```python
from build123d import *

# Parameters (mm, degrees)
F0_W     = 125
F0_H     = 95
F0_H_2   = 40
F1_DEPTH = 102
F2_START = 46
F2_DEPTH = 86.07192
F3_W     = 24
F3_H     = 50
F4_DEPTH = 3


with BuildPart() as f1:
    # F0 (on Top) → F1 (new body)
    with BuildSketch(Plane.XY):
        with Locations((62.5, 47.5)):
            Rectangle(F0_W, F0_H)
        with Locations((62.5, 115)):
            Rectangle(F0_W, F0_H_2)
    extrude(amount=F1_DEPTH)

    # F0 (on Top) → F2 (cut)
    with BuildSketch(Plane.XY.offset(F2_START)):
        with Locations((62.5, 115)):
            Rectangle(F0_W, F0_H_2)
    extrude(amount=F2_DEPTH, mode=Mode.SUBTRACT)

    # F3 (on face) → F4 (join)
    with BuildSketch(Plane.XZ):
        with Locations((15.6, 48)):
            Rectangle(F3_W, F3_H)
    extrude(amount=F4_DEPTH)


solid = f1.part
```
Can you work these out from the model? Positions are in its coordinate system, mm. A direction names the side the tool comes from. Round coordinates to 2 decimals unless told otherwise and drop trailing zeros. Loops run counter-clockwise (first coordinate to the right, second up) from the corner with the lowest first, then second, coordinate; pieces in that order, holes last. Notation, with made-up numbers: (67, 58.25) -> (112, 58.25) arc R15 cw to (112, 71.25) -> close; hole circle Ø10 at (-22.75, 52). An arc over 180 degrees is marked (long way). One line per item, written item: value. Start each with the question number.
1. If we section it at A-A, the plane x = 10: Write out the boundary of the cut face in (y, z).
2. For faces 1 (the flat face through (62, 115, 46)), 2 (the flat face through (62, 68, 0)), which set-ups out of +Z, -Z, +X, -X, +Y, -Y let a thin tool reach every point of the face, with its end or its side?
3. For pin 1 (1.5 mm diameter, centred on y = -1.5, z = 36.5, fed in from +X); pin 2 (6 mm diameter, centred on y = 70, z = 22.5, fed in from -X); pin 3 (3.5 mm diameter, centred on x = 10, y = -2, fed in from -Z); pin 4 (1.5 mm diameter, centred on x = 51, z = 19, fed in from -Y), each with a flat end and sliding along its axis, tell me the tip position at first contact or that it passes through.
4. If we section it at C-C, the plane x = 117.5: Write out the boundary of the cut face in (y, z).
5. If we section it at D-D, the plane y = 99: Write out the boundary of the cut face in (x, z), then the cut area to 3 significant figures.
6. If I drill on probe 1 along Y at (x, z) = (15, 63); probe 2 along Z at (x, y) = (20.5, 107); probe 3 along Y at (x, z) = (15.5, 82.5), over which ranges is the centre line in solid material (lowest first)?
7. If we section it at B-B, the plane z = 28: Write out the boundary of the cut face in (x, y).
Calculated:
1. outline: (-3, 23) -> (0, 23) -> (0, 0) -> (135, 0) -> (135, 46) -> (95, 46) -> (95, 102) -> (0, 102) -> (0, 73) -> (-3, 73) -> close
2. face 1: +Z, +X, -X, +Y
2. face 2: -Z, +X, -X, +Y, -Y
3. pin 1: stops at x = 27.6
3. pin 2: stops at x = 0
3. pin 3: stops at z = 23
3. pin 4: stops at y = 0
4. outline: (0, 0) -> (135, 0) -> (135, 46) -> (95, 46) -> (95, 102) -> (0, 102) -> close
5. outline: (0, 0) -> (125, 0) -> (125, 46) -> (0, 46) -> close
5. area: 5,750 mm²
6. probe 1: y = -3 to 95
6. probe 2: z = 0 to 46
6. probe 3: y = 0 to 95
7. outline: (0, 0) -> (3.6, 0) -> (3.6, -3) -> (27.6, -3) -> (27.6, 0) -> (125, 0) -> (125, 135) -> (0, 135) -> close
